Here's how the part is built. I have some questions about the finished solid (model axes, mm). A direction names the side the tool comes from. Coordinates: 2 decimals unless noted, no trailing zeros. Write each loop counter-clockwise with the first axis right and the second up, starting at its lowest first coordinate (ties: lowest second). Pieces come first, ordered by that corner, then holes.
```python
from build123d import *

# Parameters (mm, degrees)
SCHIZZO1_W                   = 10
SCHIZZO1_H                   = 18
ESTRUSIONE_ESTRUSIONE1_DEPTH = 0.9
SCHIZZO2_W                   = 8.2
SCHIZZO2_H                   = 13.8
ESTRUSIONE_ESTRUSIONE2_DEPTH = 1.6
RACCORDO1_R                  = 0.1
SCHIZZO3_W                   = 7
SCHIZZO3_H                   = 2
ESTRUSIONE_ESTRUSIONE3_DEPTH = 1.95
SCHIZZO4_W                   = 1.668109591
SCHIZZO4_H                   = 2
ESTRUSIONE_ESTRUSIONE4_DEPTH = 0.0001
TAGLIO_ESTRUSIONE1_DEPTH     = 0.0001


with BuildPart() as part:
    # Schizzo1 → Estrusione-Estrusione1 (new body)
    with BuildSketch(Plane(origin=(0, 0, 0), x_dir=(1, 0, 0), z_dir=(0, 1, 0))):
        with Locations((-8.221633561, 21.179815737)):
            Rectangle(SCHIZZO1_W, SCHIZZO1_H)
    extrude(amount=ESTRUSIONE_ESTRUSIONE1_DEPTH)

    # Schizzo2 → Estrusione-Estrusione2 (add)
    with BuildSketch(Plane(origin=(0, 0.9, 0), x_dir=(1, 0, 0), z_dir=(0, 1, 0))):
        with Locations((-8.221633561, 20.179815737)):
            Rectangle(SCHIZZO2_W, SCHIZZO2_H)
    extrude(amount=ESTRUSIONE_ESTRUSIONE2_DEPTH)

    # Raccordo1
    raccordo1_edges = [part.edges().sort_by_distance(p)[0] for p in [
        (-12.321633561, 1.7, -27.079815737),
        (-12.321633561, 1.7, -13.279815737),
        (-4.121633561, 1.7, -13.279815737),
        (-4.121633561, 1.7, -27.079815737),
        (-12.321633561, 2.5, -20.179815737),
        (-8.221633561, 2.5, -13.279815737),
        (-4.121633561, 2.5, -20.179815737),
        (-8.221633561, 2.5, -27.079815737),
    ]]
    fillet(raccordo1_edges, radius=RACCORDO1_R)

    # Schizzo3 → Estrusione-Estrusione3 (add)
    with BuildSketch(Plane(origin=(0, 0.9, 0), x_dir=(1, 0, 0), z_dir=(0, 1, 0))):
        with Locations((-9.121633561, 28.679815737)):
            Rectangle(SCHIZZO3_W, SCHIZZO3_H)
    extrude(amount=ESTRUSIONE_ESTRUSIONE3_DEPTH)

    # Schizzo4 → Estrusione-Estrusione4 (add)
    with BuildSketch(Plane(origin=(0, 2.85, 0), x_dir=(1, 0, 0), z_dir=(0, 1, 0))):
        with Locations((-6.455688357, 28.679815737)):
            Rectangle(SCHIZZO4_W, SCHIZZO4_H)
    extrude(amount=ESTRUSIONE_ESTRUSIONE4_DEPTH)

    # Schizzo6 → Taglio-Estrusione1 (cut)
    # profile 1 of 3: a face of its own
    with BuildSketch(Plane(origin=(0, 2.5, 0), x_dir=(1, 0, 0), z_dir=(0, 1, 0))):
        with BuildLine():
            Line((-8.721633561, 23.545200352), (-8.721633561, 22.862307724))
            add(Edge.make_bspline(
                [(-8.721633561, 22.862307724), (-8.721809311, 22.828879246), (-8.722149959, 22.764086535), (-8.72743309, 22.669867093), (-8.73463676, 22.581618283), (-8.746066853, 22.49931451), (-8.75985863, 22.422993808), (-8.776560446, 22.352426171), (-8.79658706, 22.287835998), (-8.828433341, 22.210723262), (-8.875756509, 22.122802601), (-8.945685074, 22.027604208), (-9.031217538, 21.946199969), (-9.127700193, 21.876013652), (-9.233835965, 21.820212532), (-9.347095154, 21.779843235), (-9.466016895, 21.75428536), (-9.547660073, 21.751656925), (-9.588921221, 21.750328557)],
                knots=[0, 0, 0, 0, 1.001505555, 1.941167018, 2.826882275, 3.653841531, 4.429895133, 5.150066043, 5.825578002, 6.45369114, 7.647487171, 8.808567382, 9.977351308, 11.170798116, 12.373658725, 13.556498008, 14.765093433, 16, 16, 16, 16], degree=3))
            add(Edge.make_bspline(
                [(-9.588921221, 21.750328557), (-9.627580326, 21.751400647), (-9.703549112, 21.753507404), (-9.814482881, 21.774339057), (-9.920517432, 21.805354415), (-10.020345579, 21.850379552), (-10.112684314, 21.908295812), (-10.196984871, 21.977991345), (-10.271204297, 22.060972988), (-10.31252402, 22.12324465), (-10.333512567, 22.154875833)],
                knots=[0, 0, 0, 0, 1.044266239, 2.052081639, 3.041743201, 4.026043445, 5.00270663, 5.980942822, 6.97441044, 8, 8, 8, 8], degree=3))
            add(Edge.make_bspline(
                [(-10.333512567, 22.154875833), (-10.348765786, 22.115108746), (-10.377948973, 22.039024459), (-10.429825242, 21.934247144), (-10.485612511, 21.843612441), (-10.546857455, 21.767020589), (-10.613698528, 21.702503806), (-10.684797277, 21.644566395), (-10.763653991, 21.596027836), (-10.848023281, 21.554329121), (-10.937313, 21.52151267), (-11.031114793, 21.498292878), (-11.128379786, 21.484025445), (-11.194675763, 21.482079939), (-11.228143977, 21.481097788)],
                knots=[0, 0, 0, 0, 1.272302504, 2.434229863, 3.488457646, 4.447234501, 5.35599188, 6.26022912, 7.18267843, 8.11661068, 9.06895546, 10.019249207, 11.000057067, 12, 12, 12, 12], degree=3))
            add(Edge.make_bspline(
                [(-11.228143977, 21.481097788), (-11.262310656, 21.48207494), (-11.329534553, 21.483997516), (-11.428292454, 21.498173108), (-11.522657231, 21.522198308), (-11.613299831, 21.555210245), (-11.699707184, 21.598539779), (-11.78296147, 21.650133961), (-11.860844851, 21.712930621), (-11.93520948, 21.782926386), (-12.002032852, 21.862204121), (-12.061524209, 21.947726181), (-12.110674198, 22.040722655), (-12.151445315, 22.139751415), (-12.183042722, 22.245470508), (-12.204979107, 22.357487955), (-12.219794287, 22.475828098), (-12.221010067, 22.557038433), (-12.221633561, 22.598685929)],
                knots=[0, 0, 0, 0, 0.978404568, 1.925038397, 2.85041836, 3.763147166, 4.682162379, 5.614488577, 6.562659439, 7.54271123, 8.535210642, 9.526693784, 10.520907202, 11.541451354, 12.589717429, 13.675358278, 14.807842563, 16, 16, 16, 16], degree=3))
            Line((-12.221633561, 22.598685929), (-12.221633561, 23.545200352))
            Line((-12.221633561, 23.545200352), (-8.721633561, 23.545200352))
        make_face()
        with BuildLine():
            Line((-9.08060792, 23.231097788), (-10.202402792, 23.231097788))
            Line((-10.202402792, 23.231097788), (-10.202402792, 23.020060128))
            add(Edge.make_bspline(
                [(-10.202402792, 23.020060128), (-10.202006197, 22.989211054), (-10.201239894, 22.929604358), (-10.198975616, 22.843055067), (-10.192913178, 22.762917749), (-10.18650115, 22.688916263), (-10.176627939, 22.621546602), (-10.164545903, 22.560583229), (-10.151879752, 22.505478502), (-10.130278548, 22.441959534), (-10.098677918, 22.369929866), (-10.048483138, 22.293631553), (-9.990321552, 22.225276288), (-9.921972987, 22.168200505), (-9.847351496, 22.121103006), (-9.766450427, 22.08967218), (-9.68242813, 22.067378707), (-9.624594659, 22.065423715), (-9.595231317, 22.064431121)],
                knots=[0, 0, 0, 0, 1.156481963, 2.23455883, 3.244418989, 4.168404366, 5.01828131, 5.794834307, 6.498111525, 7.13526334, 8.307595709, 9.435046769, 10.546766856, 11.659452936, 12.760769924, 13.837671619, 14.902137667, 16, 16, 16, 16], degree=3))
            add(Edge.make_bspline(
                [(-9.595231317, 22.064431121), (-9.575796396, 22.064927559), (-9.537672677, 22.065901376), (-9.482311145, 22.074764266), (-9.429577332, 22.087624406), (-9.38068408, 22.107715868), (-9.334241704, 22.132010599), (-9.292313019, 22.163613634), (-9.252600923, 22.199304177), (-9.216563546, 22.241219245), (-9.184273914, 22.289155884), (-9.155861871, 22.343570841), (-9.133449638, 22.405113859), (-9.113344673, 22.47238952), (-9.099394018, 22.546474511), (-9.087729412, 22.626644921), (-9.08179997, 22.713580859), (-9.081014133, 22.773725786), (-9.08060792, 22.804815737)],
                knots=[0, 0, 0, 0, 0.911752476, 1.788502045, 2.626783689, 3.45400582, 4.26402138, 5.080402872, 5.911472738, 6.767166405, 7.66795952, 8.620018292, 9.640966946, 10.73819047, 11.913090943, 13.176185384, 14.540321519, 16, 16, 16, 16], degree=3))
            Line((-9.08060792, 22.804815737), (-9.08060792, 23.231097788))
        make_face(mode=Mode.SUBTRACT)
        with BuildLine():
            Line((-10.561377151, 23.231097788), (-11.862659202, 23.231097788))
            Line((-11.862659202, 23.231097788), (-11.862659202, 22.783782083))
            add(Edge.make_bspline(
                [(-11.862659202, 22.783782083), (-11.862276795, 22.751762998), (-11.861539755, 22.690050433), (-11.859107362, 22.600951316), (-11.853690782, 22.518592948), (-11.844860313, 22.442927938), (-11.835684686, 22.373290226), (-11.822985174, 22.310371666), (-11.808547365, 22.254075798), (-11.786204171, 22.188807607), (-11.751552873, 22.115264242), (-11.698965819, 22.036065441), (-11.637141399, 21.964948169), (-11.564685457, 21.905248782), (-11.486498476, 21.855951368), (-11.402989401, 21.821376216), (-11.316705845, 21.799144888), (-11.257724028, 21.796517844), (-11.228143977, 21.795200352)],
                knots=[0, 0, 0, 0, 1.159821618, 2.235403267, 3.228114831, 4.14795534, 4.994323282, 5.771256229, 6.471395042, 7.097801288, 8.267864287, 9.404187171, 10.531774336, 11.667624178, 12.792825787, 13.866573821, 14.930062559, 16, 16, 16, 16], degree=3))
            add(Edge.make_bspline(
                [(-11.228143977, 21.795200352), (-11.209648244, 21.795469643), (-11.172955116, 21.796003882), (-11.119074178, 21.804363823), (-11.066648588, 21.816026487), (-11.016471096, 21.832915026), (-10.967725208, 21.854210104), (-10.921260001, 21.880934621), (-10.875964474, 21.911796374), (-10.818766488, 21.960074353), (-10.752842263, 22.030229244), (-10.688307172, 22.129941735), (-10.636258684, 22.243312419), (-10.614159305, 22.325540142), (-10.602743336, 22.368016858)],
                knots=[0, 0, 0, 0, 0.723503378, 1.435336582, 2.130201219, 2.824764462, 3.504949994, 4.209866579, 4.920640069, 5.648298893, 7.13757748, 8.670694625, 10.280166878, 12, 12, 12, 12], degree=3))
            add(Edge.make_bspline(
                [(-10.602743336, 22.368016858), (-10.59928802, 22.385045938), (-10.591796182, 22.421968496), (-10.583892945, 22.482176382), (-10.576803483, 22.551142736), (-10.571697091, 22.628572782), (-10.566215467, 22.714774469), (-10.564159524, 22.809720106), (-10.561650137, 22.913476814), (-10.561470474, 22.985469274), (-10.561377151, 23.022864615)],
                knots=[0, 0, 0, 0, 0.634452549, 1.375623993, 2.216454381, 3.166361212, 4.209414599, 5.370755378, 6.634280627, 8, 8, 8, 8], degree=3))
            Line((-10.561377151, 23.022864615), (-10.561377151, 23.231097788))
        make_face(mode=Mode.SUBTRACT)
    # profile 2 of 3: a face of its own
    with BuildSketch(Plane(origin=(0, 2.5, 0), x_dir=(1, 0, 0), z_dir=(0, 1, 0))):
        Polygon((-8.721633561, 20.76314907), (-8.721633561, 20.449046506), (-11.862659202, 20.449046506), (-11.862659202, 19.10289266), (-12.221633561, 19.10289266), (-12.221633561, 20.76314907), align=None)
    # profile 3 of 3: a face of its own
    with BuildSketch(Plane(origin=(0, 2.5, 0), x_dir=(1, 0, 0), z_dir=(0, 1, 0))):
        Polygon((-8.721633561, 18.519559326), (-8.721633561, 16.545200352), (-9.08060792, 16.545200352), (-9.08060792, 18.205456762), (-10.157530997, 18.205456762), (-10.157530997, 16.545200352), (-10.516505356, 16.545200352), (-10.516505356, 18.205456762), (-11.862659202, 18.205456762), (-11.862659202, 16.545200352), (-12.221633561, 16.545200352), (-12.221633561, 18.519559326), align=None)
    extrude(amount=-TAGLIO_ESTRUSIONE1_DEPTH, mode=Mode.SUBTRACT)


solid = part.part
```
1) Will these pins go through, and if not, where does the flat tip stop? pin 1 (3 mm diameter, centred on x = -9, z = -20, fed in from +Y); pin 2 (1.5 mm diameter, centred on y = 2, z = -28, fed in from +X); pin 3 (2 mm diameter, centred on x = -11, z = -25, fed in from -Y); pin 4 (1.6 mm diameter, centred on x = -10, y = 2, fed in from -Z).
Values follow:
pin 1: stops at y = 2.5
pin 2: stops at x = -5.62
pin 3: stops at y = 0
pin 4: stops at z = -29.68
2) I need wall thicknesses on probe 1 along Z at (x, y) = (-6.75, 1.95); probe 2 along Y at (x, z) = (-6, -17.5); probe 3 along X at (y, z) = (1.35, -24.25). Which ranges of each line are inside material? Lowest first, please.
Values follow:
probe 1: z = -29.68 to -27.68, -27.08 to -13.28
probe 2: y = 0 to 2.5
probe 3: x = -12.32 to -4.12
3) We'd pull the mould along Z, two halves only. Please class faces 6 (the face through (-8, 2, -27.08)), 7 (the face through (-13.222, 0.4, -21.1)), 8 (the face through (-8, 2, -13.28)): pulls with the +Z half, pulls with the -Z half, needs draft (parallel to the pull), parting line crosses it, or undercut.
Values follow:
face 6: undercut
face 7: needs draft
face 8: pulls with the +Z half
4) Imagine slicing it at A-A on y = 1.4. Please give me the cut outline in (x, z), then the cut area to 3 significant figures.
Values follow:
outline: (-12.62, -29.68) - (-5.62, -29.68) - (-5.62, -27.68) - (-12.62, -27.68) - close; (-12.32, -26.98) arc R0.1 ccw to (-12.22, -27.08) - (-4.22, -27.08) arc R0.1 ccw to (-4.12, -26.98) - (-4.12, -13.38) arc R0.1 ccw to (-4.22, -13.28) - (-12.22, -13.28) arc R0.1 ccw to (-12.32, -13.38) - close
area: 127 mm2
5) Imagine slicing it at B-B on z = -24. Please give me the cut outline in (x, y).
Values follow:
outline: (-13.22, 0) - (-3.22, 0) - (-3.22, 0.9) - (-4.12, 0.9) - (-4.12, 2.4) arc R0.1 ccw to (-4.22, 2.5) - (-12.22, 2.5) arc R0.1 ccw to (-12.32, 2.4) - (-12.32, 0.9) - (-13.22, 0.9) - close
6) Imagine slicing it at C-C on x = -8. Please give me the cut outline in (y, z).
Values follow:
outline: (0, -30.18) - (0.9, -30.18) - (0.9, -29.68) - (2.85, -29.68) - (2.85, -27.68) - (0.9, -27.68) - (0.9, -27.08) - (2.4, -27.08) arc R0.1 ccw to (2.5, -26.98) - (2.5, -13.38) arc R0.1 ccw to (2.4, -13.28) - (0.9, -13.28) - (0.9, -12.18) - (0, -12.18) - close
7) On a 3-axis mill with a long thin cutter (end or side, diameter ignored), from which of +Z, -Z, +X, -X, +Y, -Y can I reach the whole of each face in a straight line? I mean faces 1 (the face through (-9, 2, -29.68)), 2 (the face through (-8, 2.5, -20)), 3 (the face through (-4.122, 2, -20)), 4 (the face through (-12.622, 2, -29)), 5 (the face through (-5.622, 2, -29)). Say none if no direction works.
Values follow:
face 1: -Z, +X, -X, +Y
face 2: +Z, +X, -X, +Y
face 3: +Z, -Z, +X, +Y
face 4: +Z, -Z, -X, +Y
face 5: -Z, +X, +Y
8) Imagine slicing it at D-D on z = -27.5. Please give me the cut outline in (x, y).
Values follow:
outline: (-13.22, 0) - (-3.22, 0) - (-3.22, 0.9) - (-13.22, 0.9) - close
